```python
from build123d import *

# Parameters (mm, degrees)
SKETCH1_R           = 57.5
BOSS_EXTRUDE1_DEPTH = 30
CUT_EXTRUDE1_DEPTH  = 87.674679117


with BuildPart() as part:
    # Sketch1 → Boss-Extrude1 (new body)
    with BuildSketch(Plane(origin=(0, 0, 0), x_dir=(1, 0, 0), z_dir=(0, 1, 0))):
        with Locations(Location((0, 0, 0), (0, 0, 270))):
            Circle(SKETCH1_R)
    extrude(amount=BOSS_EXTRUDE1_DEPTH)

    # Sketch2 → Cut-Extrude1 (cut, through all)
    with BuildSketch(Plane.XZ):
        with BuildLine():
            Line((1, 1.732050808), (1, 2.5))
            Line((1, 2.5), (-1, 2.5))
            Line((-1, 2.5), (-1, 1.732050808))
            ThreePointArc((-1, 1.732050808), (0, -2), (1, 1.732050808))
        make_face()
    extrude(amount=-CUT_EXTRUDE1_DEPTH, mode=Mode.SUBTRACT)


solid = part.part
```
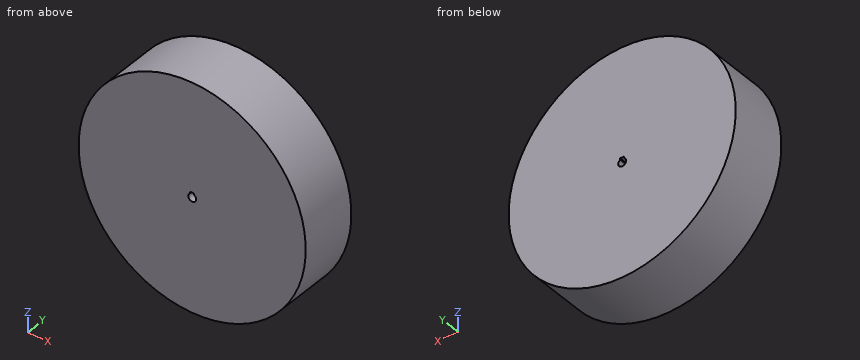
Here's how the part is built. I have some questions about the finished solid (model axes, mm). Round coordinates to 2 decimals unless told otherwise and drop trailing zeros. Write each loop counter-clockwise with the first axis right and the second up, starting at its lowest first coordinate (ties: lowest second). Pieces come first, ordered by that corner, then holes. Notation, with made-up numbers: M -24.75,44 L -15.75,44 A20 cw -15.75,76 Z; hole C 24,-2 d9. An arc over 180 degrees is marked long. Answer as CSV lines item,"result". Start each with the question number.
1. Suppose I cut it at B-B on y = 25.25. Write out the boundary of the cut face in (x, z).
2. I need wall thicknesses on probe 1 along X at (y, z) = (4.25, 46.5); probe 2 along X at (y, z) = (10, -17.5); probe 3 along Z at (x, y) = (-52, 9.75). Which ranges of each line are inside material? Lowest first, please.
3. Suppose I cut it at C-C on x = 27.5. Write out the boundary of the cut face in (y, z).
4. I'm going to push flat-ended pins straight in: pin 1 Ø6.5 at (x, z) = (0, 0) entering from +Y; pin 2 Ø1.5 at (y, z) = (16.5, 10.5) entering from +X; pin 3 Ø1 at (y, z) = (20, 5) entering from +X; pin 4 Ø4 at (x, y) = (-31, 13.5) entering from -Z. Where does each tip first touch, or does it pass through?
5. Suppose I cut it at D-D on z = -38. Write out the boundary of the cut face in (x, y).
6. Suppose I cut it at A-A on z = 0. Write out the boundary of the cut face in (x, y).
Check result:
1,outline,"C 0,0 d115; hole M -1,1.73 A2 ccw long 1,1.73 L 1,2.5 L -1,2.5 Z"
2,probe 1,"x = -33.82 to 33.82"
2,probe 2,"x = -54.77 to 54.77"
2,probe 3,"z = -24.54 to 24.54"
3,outline,"M 0,-50.5 L 30,-50.5 L 30,50.5 L 0,50.5 Z"
4,pin 1,"stops at y = 30"
4,pin 2,"stops at x = 56.67"
4,pin 3,"stops at x = 57.32"
4,pin 4,"stops at z = -49.65"
5,outline,"M -43.15,0 L 43.15,0 L 43.15,30 L -43.15,30 Z"
6,outline,"M -57.5,0 L -2,0 L -2,30 L -57.5,30 Z; M 2,0 L 57.5,0 L 57.5,30 L 2,30 Z"
